For this review, take the finished solid that the model builds, in its own axes (mm). Coordinates: 2 decimals unless noted, no trailing zeros. Loops run counter-clockwise (first coordinate to the right, second up) from the corner with the lowest first, then second, coordinate; pieces in that order, holes last. Notation, with made-up numbers: (75, 40) -> (105, 40) arc R17 ccw to (105, 46) -> close; hole circle Ø10 at (84, 79.5). An arc over 180 degrees is marked (long way). One line per item, written item: value.
from build123d import *

# Parameters (mm, degrees)
SKETCH_W            = 255
SKETCH_H            = 26.9944
SKETCH_R            = 1.75
PAD_DEPTH           = 2
SKETCH001_R         = 1.75
POCKET_DEPTH        = 2.001
LINEARPATTERN_COUNT = 13
LINEARPATTERN_PITCH = 20
SKETCH002_W         = 230.5
SKETCH002_H         = 4
PAD001_DEPTH        = 0.1


with BuildPart() as part:
    # Sketch → Pad (new body)
    with BuildSketch(Plane.XY):
        with Locations((127.5, -4.4972)):
            Rectangle(SKETCH_W, SKETCH_H)
        with Locations((7.5, 4.5)):
            Circle(SKETCH_R, mode=Mode.SUBTRACT)
    extrude(amount=PAD_DEPTH)

    # Sketch001 (on Face7 of Pad) → Pocket (cut, through all)
    with BuildSketch(Plane.XY.offset(2)):
        with Locations((7.5, 4.5)):
            Circle(SKETCH001_R)
    pocket = extrude(amount=-POCKET_DEPTH, mode=Mode.SUBTRACT)

    # LinearPattern: Pocket ×13
    with Locations(*[(i * LINEARPATTERN_PITCH, 0, 0) for i in range(1, LINEARPATTERN_COUNT)]):
        add(pocket, mode=Mode.SUBTRACT)

    # Sketch002 (on Face5 of LinearPattern) → Pad001 (join)
    with BuildSketch(Plane.XY.offset(2)):
        with Locations((127.5, -9.4986)):
            Rectangle(SKETCH002_W, SKETCH002_H)
        with Locations((127.5, -14.4958)):
            Rectangle(SKETCH002_W, SKETCH002_H)
    extrude(amount=PAD001_DEPTH)


solid = part.part
1. Take a section at A-A, the plane z = 0.5. Give the number of separate pieces and of enclosed holes in the cut face, and give its area (3 significant figures).
Return value:
separate pieces: 1
enclosed holes: 13
area: 6,760 mm2
2. Take a section at B-B, the plane x = 200. Give the boundary of the cut face in (y, z).
Return value:
outline: (-17.99, 0) -> (9, 0) -> (9, 2) -> (-7.5, 2) -> (-7.5, 2.1) -> (-11.5, 2.1) -> (-11.5, 2) -> (-12.5, 2) -> (-12.5, 2.1) -> (-16.5, 2.1) -> (-16.5, 2) -> (-17.99, 2) -> close
3. Insertion check: pin 1 Ø10 at (x, y) = (206.5, 6) entering from +Z. The pin has a flat end and moves straight along its axis. Give the tip position at first contact, or say it passes through.
Return value:
pin 1: stops at z = 2
4. To check wall thickness, follow probe 1 along Y at (x, z) = (47.5, 1.3); probe 2 along Z at (x, y) = (183.5, 1.75); probe 3 along Y at (x, z) = (148.5, 1). State the ranges of each line that lie inside material, in increasing order. Write a range as from..to.
Return value:
probe 1: y = -17.99..2.75, 6.25..9
probe 2: z = 0..2
probe 3: y = -17.99..3.06, 5.94..9
